Autodesk Inventor part; units mm, degrees
ref_plane "YZ Plane" through (0, 0, 0) normal (1, 0, 0) x (0, 1, 0)
ref_plane "XZ Plane" through (0, 0, 0) normal (0, 1, 0) x (-1, 0, 0)
ref_plane "XY Plane" through (0, 0, 0) normal (0, 0, 1) x (1, 0, 0)
sketch "Sketch1" plane through (0, 0, 0) normal (0, 0, 1) x (1, 0, 0)
  line L0 (114.2744, 165.7819) -> (114.2744, 213.4069)
  line L1 (114.2744, 213.4069) -> (349.2244, 213.4069)
  line L2 (114.2744, 213.4069) -> (349.2244, 213.4069) construction
  line L3 (349.2244, 213.4069) -> (349.2244, 165.7819)
  line L4 (139.6744, 189.5944) -> (139.6744, 169.4704)
  line L5 (139.6744, 189.5944) -> (231.7494, 189.5944)
  line L6 (139.6744, 189.5944) -> (231.7494, 189.5944) construction
  line L7 (323.8244, 189.5944) -> (323.8244, 169.4704)
  line L8 (323.8244, 189.5944) -> (231.7494, 189.5944)
  line L9 (323.8244, 189.5944) -> (231.7494, 189.5944) construction
  line L10 (231.7494, 189.5944) -> (231.7494, 175.3069)
  arc A0 (349.2244, 165.7819) -> (323.8244, 169.4704) centre (231.7494, -553.8848) ccw
  arc A1 (139.6744, 169.4704) -> (114.2744, 165.7819) centre (231.7494, -553.8848) ccw
extrude "Extrusion1" add sketch "Sketch1" along normal blind 6.35
properties part number "Skateboard Electronics Box"
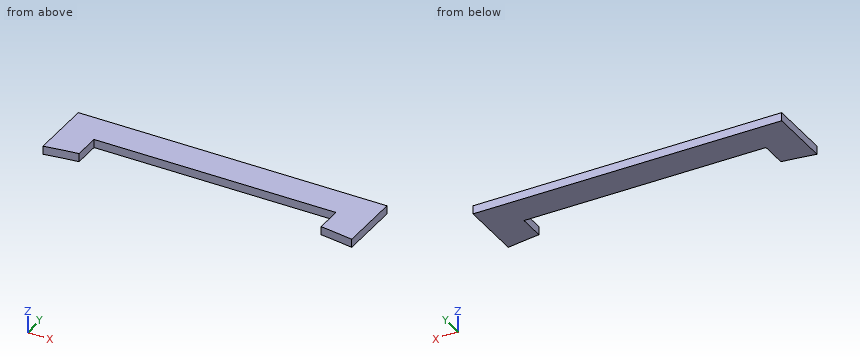
Design review of the part built by this model. Coordinates are the model's own, in mm. Coordinates: 2 decimals unless noted, no trailing zeros. Order: outer loops, then holes, each group sorted by start corner. A loop starts at its lowest first (then second) coordinate and runs counter-clockwise, first axis right, second up. Notation, with made-up numbers: M 17.25,87.5 L 61.25,87.5 A27 ccw 61.25,118.5 Z; hole C 86.25,7.5 d2. An arc over 180 degrees is marked long. Answer as a JSON object with one key per item and string values. Group by question number.
1) Add section C-C, the plane x = 232.5. Write out the cut boundary in (y, z).
2) Add section B-B, the plane z = 3.5. Write out the cut boundary in (x, y).
3) Wall thickness on L1, parallel to X at y = 174.5, z = 0.5; L2, parallel to Y at x = 156, z = 1.5; L3, parallel to Y at x = 331, z = 3: over which ranges is each line inside the solid? List them lowest first.
4) For pin 1 (1.9 mm diameter, centred on x = 201, z = 4.5, fed in from -Y), flat-tipped, find the tip position at first contact; note if it passes through.
5) Add section A-A, the plane y = 183. Write out the cut boundary in (x, z).
6) Add section D-D, the plane x = 334.5. Write out the cut boundary in (y, z).
Computed values:
{
 "1": {"outline": "M 189.59,0 L 213.41,0 L 213.41,6.35 L 189.59,6.35 Z"},
 "2": {"outline": "M 114.27,165.78 A729.16 cw 139.67,169.47 L 139.67,189.59 L 323.82,189.59 L 323.82,169.47 A729.23 cw 349.22,165.78 L 349.22,213.41 L 114.27,213.41 Z"},
 "3": {"L1": "x = 114.27 to 139.67, 323.82 to 349.22", "L2": "y = 189.59 to 213.41", "L3": "y = 168.52 to 213.41"},
 "4": {"pin 1": "stops at y = 189.59"},
 "5": {"outline": "M 114.27,0 L 139.67,0 L 139.67,6.35 L 114.27,6.35 Z; M 323.82,0 L 349.22,0 L 349.22,6.35 L 323.82,6.35 Z"},
 "6": {"outline": "M 168.03,0 L 213.41,0 L 213.41,6.35 L 168.03,6.35 Z"}
}
